```python
from build123d import *

# Parameters (mm, degrees)
F0_W     = 199.582144
F0_H     = 111.60066
F1_DEPTH = 5


with BuildPart() as f1:
    # F0 (on Front) → F1 (new body)
    with BuildSketch(Plane.XZ):
        Rectangle(F0_W, F0_H)
        Polygon((92.410073, -48.124097), (-64.657532, -48.124097), (-55.142638, -43.583292), (92.410073, -43.583292), align=None, mode=Mode.SUBTRACT)
        Polygon((92.410073, -32.43614), (92.410073, -38.146261), (-43.749776, -38.146261), (-31.784674, -32.43614), align=None, mode=Mode.SUBTRACT)
        Polygon((92.410073, -19.095723), (92.410073, -25.732951), (-17.73868, -25.732951), (-3.830899, -19.095723), align=None, mode=Mode.SUBTRACT)
        Polygon((92.410073, -5.623395), (92.410073, -11.581782), (11.91396, -11.581782), (24.399283, -5.623395), align=None, mode=Mode.SUBTRACT)
        Polygon((-92.410073, -23.323948), (-92.410073, 48.124097), (-86.056881, 48.124097), (-86.056881, -20.511512), align=None, mode=Mode.SUBTRACT)
        Polygon((-80.595024, -18.093653), (-80.595024, 48.124097), (-74.636638, 48.124097), (-74.636638, -15.45599), align=None, mode=Mode.SUBTRACT)
        Polygon((-67.933455, -12.488619), (-67.933455, 48.124097), (-62.719867, 48.124097), (-62.719867, -10.180664), align=None, mode=Mode.SUBTRACT)
        Polygon((-57.009745, -7.652903), (-57.009745, 48.124097), (-50.554827, 48.124097), (-50.554827, -4.795435), align=None, mode=Mode.SUBTRACT)
        Polygon((-90.079022, -44.876456), (-90.079022, -24.949197), (69.316997, 45.612357), (89.457676, 45.612357), (89.457676, 27.819769), (-62.871436, -44.876456), align=None, mode=Mode.SUBTRACT)
        Polygon((-43.355107, -1.608257), (-43.355107, 48.124097), (-37.893251, 48.124097), (-37.893251, 0.809602), align=None, mode=Mode.SUBTRACT)
        Polygon((-31.6866, 3.557166), (-31.6866, 48.124097), (-25.728211, 48.124097), (-25.728211, 6.194831), align=None, mode=Mode.SUBTRACT)
        Polygon((-19.025026, 9.162202), (-19.025026, 48.124097), (-12.818373, 48.124097), (-12.818373, 11.909768), align=None, mode=Mode.SUBTRACT)
        Polygon((-7.356516, 14.327627), (-7.356516, 48.124097), (-2.142929, 48.124097), (-2.142929, 16.635582), align=None, mode=Mode.SUBTRACT)
        Polygon((92.410073, 6.541645), (92.410073, 0), (36.182657, 0), (49.89015, 6.541645), align=None, mode=Mode.SUBTRACT)
        Polygon((92.410073, 17.465357), (92.410073, 13.244831), (63.936138, 13.244831), (72.779912, 17.465357), align=None, mode=Mode.SUBTRACT)
        Polygon((3.81546, 19.273246), (3.81546, 48.124097), (9.277313, 48.124097), (9.277313, 21.691103), align=None, mode=Mode.SUBTRACT)
        Polygon((15.483965, 24.438669), (15.483965, 48.124097), (20.945825, 48.124097), (20.945825, 26.856529), align=None, mode=Mode.SUBTRACT)
        Polygon((26.407678, 29.274386), (26.407678, 48.124097), (30.13167, 48.124097), (30.13167, 30.922926), align=None, mode=Mode.SUBTRACT)
        Polygon((34.848724, 33.011075), (34.848724, 48.124097), (38.820986, 48.124097), (38.820986, 34.769519), align=None, mode=Mode.SUBTRACT)
        Polygon((43.289777, 36.747767), (43.289777, 48.124097), (47.5103, 48.124097), (47.5103, 38.616112), align=None, mode=Mode.SUBTRACT)
        Polygon((51.730823, 40.484456), (51.730823, 48.124097), (55.951346, 48.124097), (55.951346, 42.3528), align=None, mode=Mode.SUBTRACT)
        Polygon((60.171869, 44.221145), (60.171869, 48.124097), (68.988499, 48.124097), align=None, mode=Mode.SUBTRACT)
    extrude(amount=F1_DEPTH)


solid = f1.part
```
Could you check a few things on this model? Use its own coordinates, in mm. A direction names the side the tool comes from. Coordinates: 2 decimals unless noted, no trailing zeros. Write each loop counter-clockwise with the first axis right and the second up, starting at its lowest first coordinate (ties: lowest second). Pieces come first, ordered by that corner, then holes. Notation, with made-up numbers: (87, -28) -> (131, -28) arc R23 cw to (131, 3) -> close; hole circle Ø10 at (13, -22.5). An arc over 180 degrees is marked (long way). One line per question, with ' | ' between items. Start each with the question number.
1. If we section it at A-A (x = -48.5): Please give me the cut outline in (y, z).
2. If we section it at C-C (y = -2.65): Count the separate pieces of the cut face and the enclosed holes in it, and give its area (3 significant figures).
3. For faces 5 (the face through (-89, -2, 48.124)), 6 (the face through (-1, -5, 26)), which set-ups out of +Z, -Z, +X, -X, +Y, -Y let a thin tool reach every point of the face, with its end or its side?
4. Thinking about a two-plate mould opening in X: for faces 1 (the face through (99.791, -2, -1)), 2 (the face through (-57.01, -2, 20)), 3 (the face through (18, -2, 48.124)), 4 (the face through (-1, 0, 26)), which applies, pulls with the +X half, pulls with the -X half, needs draft (parallel to the pull), parting line crosses it, or undercut?
5. Please list where these lines run through material, in increasing order: line 1 along Z through (x, y) = (13, -4.05); line 2 along X through (y, z) = (-2, -34); line 3 along Z through (x, y) = (-65.5, -0.9).
6. If we section it at B-B (x = 41): Please give me the cut outline in (y, z).
Return value:
1) outline: (-5, -55.8) -> (0, -55.8) -> (0, -48.12) -> (-5, -48.12) -> close; (-5, -43.58) -> (0, -43.58) -> (0, -38.02) -> (-5, -38.02) -> close; (-5, -6.54) -> (0, -6.54) -> (0, 55.8) -> (-5, 55.8) -> close
2) separate pieces: 1 | enclosed holes: 22 | area: 11,300 mm²
3) face 5: +Y, -Y | face 6: +Z, -Z, +X, -X, -Y
4) face 1: pulls with the +X half | face 2: undercut | face 3: undercut | face 4: needs draft
5) line 1: z = -55.8 to -48.12, -43.58 to -38.15, -32.44 to -25.73, -19.1 to -11.58, -11.06 to -8.67, 20.68 to 55.8 | line 2: x = -99.79 to -90.08, -40.08 to -35.06, 92.41 to 99.79 | line 3: z = -55.8 to -44.88, -14.07 to -11.41, 48.12 to 55.8
6) outline: (-5, -55.8) -> (0, -55.8) -> (0, -48.12) -> (-5, -48.12) -> close; (-5, -43.58) -> (0, -43.58) -> (0, -38.15) -> (-5, -38.15) -> close; (-5, -32.44) -> (0, -32.44) -> (0, -25.73) -> (-5, -25.73) -> close; (-5, -19.1) -> (0, -19.1) -> (0, -11.58) -> (-5, -11.58) -> close; (-5, -5.62) -> (0, -5.62) -> (0, 0) -> (-5, 0) -> close; (-5, 2.3) -> (0, 2.3) -> (0, 4.69) -> (-5, 4.69) -> close; (-5, 33.08) -> (0, 33.08) -> (0, 55.8) -> (-5, 55.8) -> close
